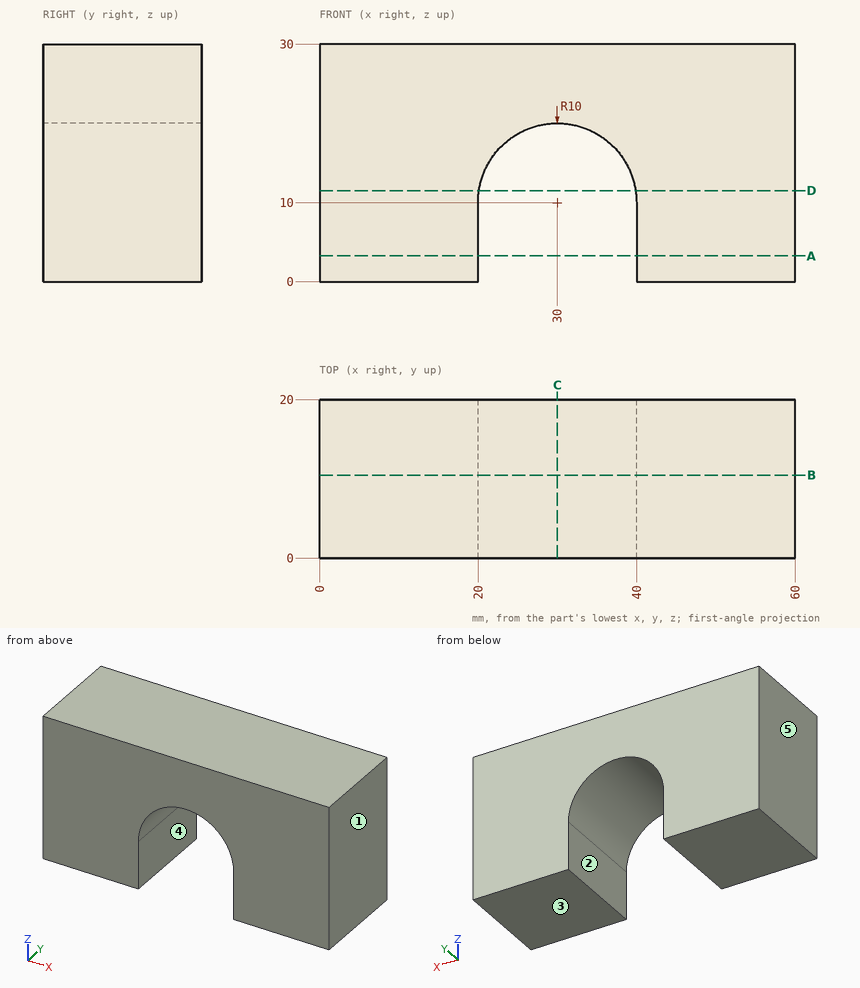
Study the drawing (mm; zero at the part's minimum x, y, z) and answer. A direction names the side the tool comes from. Round coordinates to 2 decimals unless told otherwise and drop trailing zeros. Loops run counter-clockwise (first coordinate to the right, second up) from the corner with the lowest first, then second, coordinate; pieces in that order, holes last. Notation, with made-up numbers: M -29,46 L -24,46 A14 cw -24,60 Z; hole C 43,-36 d6. An arc over 180 degrees is marked long. One line per question, with ' | ' between items.
Q1. Find section D-D, the plane z = 11.5. Give the vertices of the cut face in (x, y), then the cut area to 3 significant figures.
Conclusion:
outline: M 0,0 L 20.11,0 L 20.11,20 L 0,20 Z; M 39.89,0 L 60,0 L 60,20 L 39.89,20 Z | area: 805 mm2
Q2. Consider line 1 along X through (y, z) = (18.75, 7.75); line 2 along X through (y, z) = (16, 16.5); line 3 along Z through (x, y) = (36, 10.75). Determine where each line is inside the solid, lowest interval first. Write a range as from..to.
Conclusion:
line 1: x = 0..20, 40..60 | line 2: x = 0..22.4, 37.6..60 | line 3: z = 18..30
Q3. The mould has two halves that part along X. Classify the marked faces 3, 4 and 5: +X half, -X half, draft (parallel to the pull), parting line (faces both ways), or undercut.
Conclusion:
face 3: draft | face 4: undercut | face 5: -X half
Q4. Find section A-A, the plane z = 3.25. Give the vertices of the cut face in (x, y), then the cut area to 3 significant figures.
Conclusion:
outline: M 0,0 L 20,0 L 20,20 L 0,20 Z; M 40,0 L 60,0 L 60,20 L 40,20 Z | area: 800 mm2
Q5. Find section B-B, the plane y = 10.5. Give the vertices of the cut face in (x, z), then the cut area to 3 significant figures.
Conclusion:
outline: M 0,0 L 20,0 L 20,10 A10 cw 40,10 L 40,0 L 60,0 L 60,30 L 0,30 Z | area: 1,440 mm2
Q6. A tool of negligible diameter and unlimited length cuts with its end or side. For the marked faces 1 and 2, from which of +Z, -Z, +X, -X, +Y, -Y can it reach the whole face along a straight path? Write none if from no direction.
Conclusion:
face 1: +Z, -Z, +X, +Y, -Y | face 2: -Z, +Y, -Y
Q7. Find section C-C, the plane x = 30. Give the vertices of the cut face in (y, z), then the cut area to 3 significant figures.
Conclusion:
outline: M 0,20 L 20,20 L 20,30 L 0,30 Z | area: 200 mm2
